The model under review builds one solid part; all positions refer to its coordinate system, in mm. A direction names the side the tool comes from. Round coordinates to 2 decimals unless told otherwise and drop trailing zeros. Order: outer loops, then holes, each group sorted by start corner. A loop starts at its lowest first (then second) coordinate and runs counter-clockwise, first axis right, second up. Notation, with made-up numbers: M 1.5,33.25 L 51.5,33.25 A13 cw 51.5,56.25 Z; hole C -5,35.5 d1. An arc over 180 degrees is marked long. Answer as a JSON object with one key per item and string values. Group by question number.
1) To check wall thickness, follow line 1 (Y direction, x = 67.31, z = 1.95); line 2 (X direction, y = 26, z = 2.6); line 3 (X direction, y = -1, z = 2.35). State the ranges of each line that lie inside material, in increasing order.
2) Consider section A-A, the plane y = 21.59. Write out the cut boundary in (x, z).
3) Consider section C-C, the plane x = -64. Write out the cut boundary in (y, z).
4) The part is to be moulded in two halves that separate along Y. For faces 1 (the cylindrical face through (-99.79, -55.24, 1.42)), 2 (the cylindrical face through (99.69, 55.34, 1.42)), 3 (the cylindrical face through (-39.683, 21.799, 1.417)), say which applies: +Y half, -Y half, draft (parallel to the pull), parting line (faces both ways), or undercut.
5) Consider section B-B, the plane y = 44.45. Write out the cut boundary in (x, z) (3 decimals).
6) Consider section D-D, the plane z = 1. Count the separate pieces of the cut face and the enclosed holes in it, then the cut area to 3 significant figures.
7) For faces 4 (the cylindrical face through (77.03, 7.3, 1.38)), 5 (the cylindrical face through (-99.79, 55.24, 1.42)), list the 3-axis set-ups (+Z, -Z, +X, -X, +Y, -Y) from which the entire face can be reached by the end or side of a thin tool; tool diameter is ignored.
```python
from build123d import *

# Parameters (mm, degrees)
SKETCH1_W                       = 203.2
SKETCH1_H                       = 114.3
BOSS_EXTRUDE1_DEPTH             = 2.794
F_5_32_0_15625_DIAMETER_HOLE1_D = 3.96875
FILLET2_R                       = 6.35
SKETCH7_R                       = 8.89
SKETCH7_R_2                     = 1.5875
SKETCH7_W                       = 14.732
SKETCH7_H                       = 12.7
CUT_EXTRUDE1_DEPTH              = 117.603983362
FILLET3_R                       = 1.27
F_3_8_0_375_DIAMETER_HOLE1_D    = 9.525
SKETCH12_R                      = 1.7
CUT_EXTRUDE4_DEPTH              = 117.603983362
CUT_EXTRUDE5_DEPTH              = 117.603983362


with BuildPart() as part:
    # Sketch1 → Boss-Extrude1 (new body)
    with BuildSketch(Plane.XY):
        Rectangle(SKETCH1_W, SKETCH1_H)
    extrude(amount=BOSS_EXTRUDE1_DEPTH)

    # 5/32 (0.15625) Diameter Hole1 (through all)
    with Locations(Plane.XY.offset(2.794)):
        with Locations((95.25, -17.78), (-95.25, 50.8), (95.25, 50.8), (95.25, -50.8), (-95.25, -50.8), (-95.25, -17.78)):
            Hole(F_5_32_0_15625_DIAMETER_HOLE1_D / 2)

    # Fillet2
    fillet2_edges = [part.edges().sort_by_distance(p)[0] for p in [
        (101.6, -57.15, 1.397),
        (-101.6, -57.15, 1.397),
        (-101.6, 57.15, 1.397),
        (101.6, 57.15, 1.397),
    ]]
    fillet(fillet2_edges, radius=FILLET2_R)

    # Sketch7 → Cut-Extrude1 (cut, through all)
    with BuildSketch(Plane(origin=(0, 0, 0), x_dir=(-1, 0, 0), z_dir=(0, 0, -1))):
        with Locations((44.45, -6.35)):
            Circle(SKETCH7_R)
        with Locations((53.6, 2.8)):
            Circle(SKETCH7_R_2)
        with Locations(Location((35.3, 2.8, 0), (0, 0, 180))):
            Circle(SKETCH7_R_2)
        with Locations(Location((53.6, -15.5, 0), (0, 0, 180))):
            Circle(SKETCH7_R_2)
        with Locations((35.3, -15.5)):
            Circle(SKETCH7_R_2)
        with Locations((-15.494, -36.83)):
            Rectangle(SKETCH7_W, SKETCH7_H)
    extrude(amount=-CUT_EXTRUDE1_DEPTH, mode=Mode.SUBTRACT)

    # Fillet3
    fillet3_edges = [part.edges().sort_by_distance(p)[0] for p in [
        (22.86, -43.18, 1.397),
        (22.86, -30.48, 1.397),
        (8.128, -30.48, 1.397),
        (8.128, -43.18, 1.397),
    ]]
    fillet(fillet3_edges, radius=FILLET3_R)

    # 3/8 (0.375) Diameter Hole1 (through all)
    with Locations(Plane(origin=(0, 0, 0), x_dir=(-1, 0, 0), z_dir=(0, 0, -1))):
        with Locations((53.975, 21.59), (34.925, 21.59)):
            Hole(F_3_8_0_375_DIAMETER_HOLE1_D / 2)

    # Sketch12 → Cut-Extrude4 (cut, through all)
    with BuildSketch(Plane(origin=(0, 0, 0), x_dir=(-1, 0, 0), z_dir=(0, 0, -1))):
        with Locations((-67.31, -26.35)):
            Circle(SKETCH12_R)
        with Locations(Location((-67.31, 13.65, 0), (0, 0, 180))):
            Circle(SKETCH12_R)
        with BuildLine():
            Line((-73.46, 8.8), (-61.16, 8.8))
            ThreePointArc((-61.16, 8.8), (-57.624466094, 7.335533906), (-56.16, 3.8))
            Line((-56.16, 3.8), (-56.16, -16.5))
            ThreePointArc((-56.16, -16.5), (-57.624466094, -20.035533906), (-61.16, -21.5))
            Line((-61.16, -21.5), (-73.46, -21.5))
            ThreePointArc((-73.46, -21.5), (-76.995533906, -20.035533906), (-78.46, -16.5))
            Line((-78.46, -16.5), (-78.46, 3.8))
            ThreePointArc((-78.46, 3.8), (-76.995533906, 7.335533906), (-73.46, 8.8))
        make_face()
    extrude(amount=-CUT_EXTRUDE4_DEPTH, mode=Mode.SUBTRACT)

    # Sketch13 → Cut-Extrude5 (cut, through all)
    with BuildSketch(Plane(origin=(0, 0, 0), x_dir=(-1, 0, 0), z_dir=(0, 0, -1))):
        with BuildLine():
            Line((-79.375, 48.26), (-53.975, 48.26))
            ThreePointArc((-53.975, 48.26), (-50.165, 44.45), (-53.975, 40.64))
            Line((-53.975, 40.64), (-79.375, 40.64))
            ThreePointArc((-79.375, 40.64), (-83.185, 44.45), (-79.375, 48.26))
        make_face()
        with BuildLine():
            Line((79.375, 48.26), (53.975, 48.26))
            ThreePointArc((53.975, 48.26), (50.165, 44.45), (53.975, 40.64))
            Line((53.975, 40.64), (79.375, 40.64))
            ThreePointArc((79.375, 40.64), (83.185, 44.45), (79.375, 48.26))
        make_face()
        with BuildLine():
            Line((-34.925, 48.26), (-9.525, 48.26))
            ThreePointArc((-9.525, 48.26), (-5.715, 44.45), (-9.525, 40.64))
            Line((-9.525, 40.64), (-34.925, 40.64))
            ThreePointArc((-34.925, 40.64), (-38.735, 44.45), (-34.925, 48.26))
        make_face()
        with BuildLine():
            Line((34.925, 48.26), (9.525, 48.26))
            ThreePointArc((9.525, 48.26), (5.715, 44.45), (9.525, 40.64))
            Line((9.525, 40.64), (34.925, 40.64))
            ThreePointArc((34.925, 40.64), (38.735, 44.45), (34.925, 48.26))
        make_face()
    extrude(amount=-CUT_EXTRUDE5_DEPTH, mode=Mode.SUBTRACT)


solid = part.part
```
Results list:
{
 "1": {"line 1": "-57.15 to -28.05, -24.65 to -21.5, 8.8 to 11.95, 15.35 to 40.64, 48.26 to 57.15", "line 2": "-101.6 to -55.77, -52.18 to -36.72, -33.13 to 101.6", "line 3": "-101.6 to -51.55, -37.35 to 56.16, 78.46 to 101.6"},
 "2": {"outline": "M -101.6,0 L -58.74,0 L -58.74,2.79 L -101.6,2.79 Z; M -49.21,0 L -39.69,0 L -39.69,2.79 L -49.21,2.79 Z; M -30.16,0 L 101.6,0 L 101.6,2.79 L -30.16,2.79 Z"},
 "3": {"outline": "M -57.15,0 L 40.64,0 L 40.64,2.79 L -57.15,2.79 Z; M 48.26,0 L 57.15,0 L 57.15,2.79 L 48.26,2.79 Z"},
 "4": {"face 1": "-Y half", "face 2": "+Y half", "face 3": "undercut"},
 "5": {"outline": "M -101.6,0 L -83.185,0 L -83.185,2.794 L -101.6,2.794 Z; M -50.165,0 L -38.735,0 L -38.735,2.794 L -50.165,2.794 Z; M -5.715,0 L 5.715,0 L 5.715,2.794 L -5.715,2.794 Z; M 38.735,0 L 50.165,0 L 50.165,2.794 L 38.735,2.794 Z; M 83.185,0 L 101.6,0 L 101.6,2.794 L 83.185,2.794 Z"},
 "6": {"separate pieces": "1", "enclosed holes": "21", "area": "20,900 mm^2"},
 "7": {"face 4": "+Z, -Z", "face 5": "+Z, -Z, -X, +Y"}
}
